from build123d import *

# Parameters (mm, degrees)
AUSTRAGUNG1_PITCH               = 20
AUSTRAGUNG1_HEIGHT              = 20
AUSTRAGUNG1_RADIUS              = 4
SKIZZE2_R                       = 14.681
SKIZZE3_2_R                     = 4
SCHNITT_LINEAR_AUSTRAGEN2_DEPTH = 27
SKIZZE8_W                       = 12.67071878
SKIZZE8_H                       = 12.67071878
SCHNITT_LINEAR_AUSTRAGEN3_DEPTH = 25


with BuildPart() as part:
    # Austragung1: sweep along a helix
    with BuildLine() as austragung1_path:
        Helix(AUSTRAGUNG1_PITCH, AUSTRAGUNG1_HEIGHT, AUSTRAGUNG1_RADIUS, center=(-3.071, 0, 0), direction=(0, 0, 1))
    # Skizze2 → Austragung1 (sweep)
    with BuildSketch(Plane.XY):
        Circle(SKIZZE2_R)
    sweep(path=austragung1_path.line, is_frenet=True)

    # Skizze3<2> → Schnitt-Linear austragen2 (cut)
    with BuildSketch(Plane.XY):
        with Locations(Location((-3.071, 0, 0), (0, 0, 180))):
            Circle(SKIZZE3_2_R)
    extrude(amount=SCHNITT_LINEAR_AUSTRAGEN2_DEPTH, mode=Mode.SUBTRACT)

    # Skizze8 → Schnitt-Linear austragen3 (cut)
    with BuildSketch(Plane.XY.offset(20)):
        with Locations((-3.071, 0)):
            Rectangle(SKIZZE8_W, SKIZZE8_H)
    extrude(amount=-SCHNITT_LINEAR_AUSTRAGEN3_DEPTH, mode=Mode.SUBTRACT)


solid = part.part
Source: CAD feature listing. Evaluate the final solid. Frame: model axes, mm. A direction names the side the tool comes from. Round coordinates to 2 decimals unless told otherwise and drop trailing zeros. One line per item, written item: value. Start each with the question number.
Item 1: Mould query, pull axis X, two halves, no side actions, for faces 1 (the flat face through (-3, -6.335, 10)), 2 (the flat face through (3.264, 0, 10)), 3 (the flat face through (5, 0, 0)). Classes: pulls with the +X half, pulls with the -X half, needs draft (parallel to the pull), parting line crosses it, or undercut.
Item 2: Ray query, L1, parallel to Z at x = 8, y = 11; L2, parallel to X at y = -6, z = 6.5; L3, parallel to X at y = 0.5, z = 9.5. Return the intervals inside material, ascending. Write a range as from..to.
Item 3: Pin query (flat end, axial travel): pin 1 (12 mm diameter, centred on y = 9, z = 10, fed in from -X); pin 2 (4 mm diameter, centred on x = 10, y = 13.5, fed in from +Z); pin 3 (8 mm diameter, centred on x = 2, z = 4, fed in from -Y); pin 4 (4 mm diameter, centred on x = 2.5, y = -0.5, fed in from -Z). Return the tip coordinate at first contact, or that it passes through.
Item 4: Set-up query: faces 4 (the flat face through (5, 0, 20)), 5 (the flat face through (-3, 6.335, 10)). Return all of +Z, -Z, +X, -X, +Y, -Y with unobstructed straight access to the full face (end or side cutting, diameter ignored); none if empty.
Result set:
1. face 1: undercut
1. face 2: undercut
1. face 3: needs draft
2. L1: z = 0..6.21, 18.77..20
2. L2: x = -16.26..-9.41, 3.26..7.33
2. L3: x = -20.79..-9.41, 3.26..8.58
3. pin 1: stops at x = -20.56
3. pin 2: stops at z = 4.95
3. pin 3: stops at y = -14.57
3. pin 4: stops at z = 0
4. face 4: +Z, +X, -X, +Y, -Y
4. face 5: +Z, -Z
